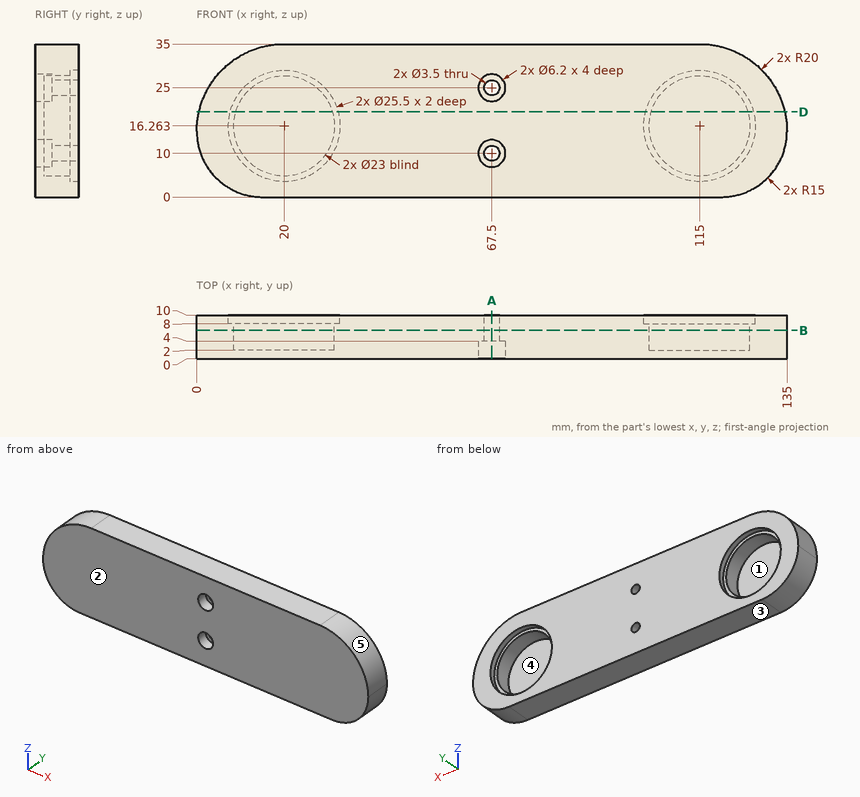
The figure shows three views and two pictorial views of one solid part (mm, origin at its lowest corner). Answer the questions. A direction names the side the tool comes from. Give positions to 0.01 mm unless a question says otherwise; leave off trailing zeros. Order: outer loops, then holes, each group sorted by start corner. A loop starts at its lowest first (then second) coordinate and runs counter-clockwise, first axis right, second up. Notation, with made-up numbers: (5, -23) -> (50, -23) arc R24 cw to (50, -9) -> close; hole circle Ø4 at (0.5, -39). An arc over 180 degrees is marked (long way). One line per item, written item: value.
1) A tool of negligible diameter and unlimited length cuts with its end or side. For the marked faces 1 and 2, from which of +Z, -Z, +X, -X, +Y, -Y can it reach the whole face along a straight path? Write none if from no direction.
Reported:
face 1: +Y
face 2: +Z, -Z, +X, -X, -Y
2) Find section D-D, the plane z = 19.5. Determine the outline of the cut face in (x, y) (1 decimal).
Reported:
outline: (0.5, 0) -> (134.5, 0) -> (134.5, 10) -> (127.3, 10) -> (127.3, 8) -> (126, 8) -> (126, 2) -> (104, 2) -> (104, 8) -> (102.7, 8) -> (102.7, 10) -> (32.3, 10) -> (32.3, 8) -> (31, 8) -> (31, 2) -> (9, 2) -> (9, 8) -> (7.7, 8) -> (7.7, 10) -> (0.5, 10) -> close
3) Find section A-A, the plane x = 67.5. Determine the outline of the cut face in (y, z), plus the area to 3 significant figures.
Reported:
outline: (0, 0) -> (10, 0) -> (10, 8.25) -> (4, 8.25) -> (4, 6.9) -> (0, 6.9) -> close; (0, 13.1) -> (4, 13.1) -> (4, 11.75) -> (10, 11.75) -> (10, 23.25) -> (4, 23.25) -> (4, 21.9) -> (0, 21.9) -> close; (0, 28.1) -> (4, 28.1) -> (4, 26.75) -> (10, 26.75) -> (10, 35) -> (0, 35) -> close
area: 258 mm^2
4) Flat-ended cylindrical pins translate along their axes: P1, Ø13, axis at x = 17.5, z = 14, coming from the +Y side; P2, Ø3, axis at x = 67.5, z = 10, coming from the -Y side; P3, Ø20.5, axis at x = 113, z = 15, coming from the +Y side; P4, Ø5.5, axis at x = 67.5, z = 10, coming from the -Y side. Find the tip coordinate at first contact, or state that the pin passes through.
Reported:
P1: stops at y = 2
P2: passes through
P3: stops at y = 8
P4: stops at y = 4
5) Find the intervals of material crossed by line 1 (Z direction, x = 67.5, y = 8.3); line 2 (X direction, y = 5.75, z = 16) (1 decimal); line 3 (X direction, y = 3.5, z = 14.5), in increasing order.
Reported:
line 1: z = 0 to 8.25, 11.75 to 23.25, 26.75 to 35
line 2: x = 0 to 8.5, 31.5 to 103.5, 126.5 to 135
line 3: x = 0.01 to 8.64, 31.36 to 103.64, 126.36 to 134.99
6) Determine the mould class of the marked faces 3, 4 and 5 for opening direction Z: pulls with the +Z half, pulls with the -Z half, needs draft (parallel to the pull), parting line crosses it, or undercut.
Reported:
face 3: pulls with the -Z half
face 4: undercut
face 5: pulls with the +Z half
7) Find section B-B, the plane y = 6.5. Count the separate pieces of the cut face and the enclosed holes in it, plus the area to 3 significant figures.
Reported:
separate pieces: 1
enclosed holes: 4
area: 3,610 mm^2
